For this review, take the finished solid that the model builds, in its own axes (mm). A direction names the side the tool comes from. Round coordinates to 2 decimals unless told otherwise and drop trailing zeros. Loops run counter-clockwise (first coordinate to the right, second up) from the corner with the lowest first, then second, coordinate; pieces in that order, holes last. Notation, with made-up numbers: (20, -36) -> (45, -36) arc R30 cw to (45, -3) -> close; hole circle Ø3 at (-9, 68). An arc over 180 degrees is marked (long way). Use one line per item in the form item = value. Start each with the question number.
from build123d import *

# Parameters (mm, degrees)
F0_R          = 20
F1_DEPTH      = 470
F1_DEPTH_BACK = 470


with BuildPart() as f1:
    # F0 (on Front) → F1 (new body, two sides)
    with BuildSketch(Plane.XZ) as f1_sk:
        with BuildLine():
            Line((-10, 234.674186), (-10, 248.989795))
            ThreePointArc((-10, 248.989795), (0, 150), (10, 248.989795))
            Line((10, 248.989795), (10, 234.674186))
            Line((10, 234.674186), (-10, 234.674186))
        make_face()
        with Locations((0, 200)):
            Circle(F0_R, mode=Mode.SUBTRACT)
    extrude(amount=F1_DEPTH)
    extrude(f1_sk.sketch, amount=-F1_DEPTH_BACK)


solid = f1.part
Item 1: Take a section at C-C on y = 393. Give the boundary of the cut face in (x, z).
Item 2: Take a section at D-D on x = -35. Give the boundary of the cut face in (y, z), plus the area to 3 significant figures.
Item 3: Draft analysis for pull direction X (two halves, no side actions). For faces 1 (the flat face through (22, 470, 200)), 2 (the cylindrical face through (-2.058, -6.58, 150.042)), 3 (the flat face through (10, -7, 242)), state which applies: +X half, -X half, draft (parallel to the pull), parting line (faces both ways), or undercut.
Item 4: Take a section at B-B on x = 0. Give the boundary of the cut face in (y, z), plus the area to 3 significant figures.
Item 5: For P1, Ø7, axis at y = -62, z = 242.5, coming from the -X side; P2, Ø6, axis at y = 90, z = 166, coming from the -X side; P3, Ø3, axis at y = -96.5, z = 204.5, coming from the +X side, all flat-tipped, find the tip position at first contact; note any pin that passes through.
Item 6: Machinability: for faces 4 (the flat face through (22, -470, 200)), 5 (the flat face through (-10, -7, 242)), which of the approach directions +Z, -Z, +X, -X, +Y, -Y give a long, thin tool a straight path to every point of the face, cutting with its end or side? Answer none if there is none.
Item 7: Take a section at A-A on z = 200. Give the boundary of the cut face in (x, y).
Item 8: Wall thickness on line 1 (Z direction, x = 0, y = 278); line 2 (Z direction, x = -9, y = 175.5); line 3 (X direction, y = -189, z = 238): over which ranges is each line inside the solid? List them lowest first.
Results:
q1.outline = (-10, 234.67) -> (-10, 248.99) arc R50 ccw (long way) to (10, 248.99) -> (10, 234.67) -> close; hole circle Ø40 at (0, 200)
q2.outline = (-470, 164.29) -> (470, 164.29) -> (470, 235.71) -> (-470, 235.71) -> close
q2.area = 67,100 mm2
q3.face_1 = draft
q3.face_2 = parting line
q3.face_3 = undercut
q4.outline = (-470, 150) -> (470, 150) -> (470, 180) -> (-470, 180) -> close; (-470, 220) -> (470, 220) -> (470, 234.67) -> (-470, 234.67) -> close
q4.area = 42,000 mm2
q5.P1 = -31.29
q5.P2 = -39.23
q5.P3 = 49.91
q6.face_4 = +Z, -Z, +X, -X, -Y
q6.face_5 = +Z, +Y, -Y
q7.outline = (-50, -470) -> (-20, -470) -> (-20, 470) -> (-50, 470) -> close; (20, -470) -> (50, -470) -> (50, 470) -> (20, 470) -> close
q8.line_1 = 150 to 180, 220 to 234.67
q8.line_2 = 150.82 to 182.14, 217.86 to 234.67
q8.line_3 = -32.5 to -10, 10 to 32.5
